```python
from build123d import *

# Parameters (mm, degrees)
SKETCH1_W           = 2.54
SKETCH1_H           = 2.54
BOSS_EXTRUDE1_DEPTH = 29.21
SKETCH2_OUTSIDE_W   = 10.426
SKETCH2_OUTSIDE_H   = 10.426
SKETCH2_OUTSIDE_W_2 = 1.905
SKETCH2_OUTSIDE_H_2 = 1.905
CUT_EXTRUDE1_DEPTH  = 11.43
FILLET1_R           = 1.27
SKETCH3_W           = 1.524
SKETCH3_H           = 16.51
BOSS_EXTRUDE2_DEPTH = 20.32
CUT_EXTRUDE2_DEPTH  = 38.147445726
CUT_EXTRUDE3_DEPTH  = 38.147445726


with BuildPart() as part:
    # Sketch1 → Boss-Extrude1 (new body)
    with BuildSketch(Plane(origin=(0, 0, 0), x_dir=(1, 0, 0), z_dir=(0, 1, 0))):
        with Locations((1.27, 1.27)):
            Rectangle(SKETCH1_W, SKETCH1_H)
    extrude(amount=BOSS_EXTRUDE1_DEPTH)

    # Sketch2 outside → Cut-Extrude1 (cut)
    with BuildSketch(Plane(origin=(0, 29.21, 0), x_dir=(1, 0, 0), z_dir=(0, 1, 0))):
        with Locations((1.27, 1.27)):
            Rectangle(SKETCH2_OUTSIDE_W, SKETCH2_OUTSIDE_H)
        with Locations((1.27, 1.27)):
            Rectangle(SKETCH2_OUTSIDE_W_2, SKETCH2_OUTSIDE_H_2, mode=Mode.SUBTRACT)
    extrude(amount=-CUT_EXTRUDE1_DEPTH, mode=Mode.SUBTRACT)

    # Fillet1
    fillet1_edges = [part.edges().sort_by_distance(p)[0] for p in [
        (1.27, 0, -2.54),
        (2.54, 0, -1.27),
        (1.27, 0, 0),
        (0, 0, -1.27),
    ]]
    fillet(fillet1_edges, radius=FILLET1_R - 0.0001)  # a hair under: the kernel refuses the full size

    # Sketch3 → Boss-Extrude2 (add)
    with BuildSketch(Plane(origin=(2.54, 0, 0), x_dir=(0, 0, -1), z_dir=(1, 0, 0))):
        with Locations((1.27, 9.525)):
            Rectangle(SKETCH3_W, SKETCH3_H)
    extrude(amount=BOSS_EXTRUDE2_DEPTH)

    # Sketch4 → Cut-Extrude2 (cut, through all)
    with BuildSketch(Plane.XY.offset(-0.508)):
        Polygon((2.54, 17.78), (22.86, 9.525), (22.86, 17.78), align=None)
    extrude(amount=-CUT_EXTRUDE2_DEPTH, mode=Mode.SUBTRACT)

    # Sketch5 → Cut-Extrude3 (cut, through all)
    with BuildSketch(Plane.XY.offset(-0.508)):
        Polygon((2.54, 1.27), (22.86, 9.525), (22.86, 1.27), align=None)
    extrude(amount=-CUT_EXTRUDE3_DEPTH, mode=Mode.SUBTRACT)


solid = part.part
```
The model under review builds one solid part; all positions refer to its coordinate system, in mm. A direction names the side the tool comes from. Round coordinates to 2 decimals unless told otherwise and drop trailing zeros. Write each loop counter-clockwise with the first axis right and the second up, starting at its lowest first coordinate (ties: lowest second). Pieces come first, ordered by that corner, then holes. Notation, with made-up numbers: (5, -39) -> (52, -39) arc R20 cw to (52, -11) -> close; hole circle Ø8 at (2.25, 81.5). An arc over 180 degrees is marked (long way). Use CSV: the item, a comma, the result in double quotes.
Q1. For faces 1 (the flat face through (1, 24, -2.222)), 2 (the flat face through (0.318, 24, -1)), 3 (the flat face through (10, 9, -0.508)), 4 (the flat face through (2.54, 9.41, -2.38)), list the 3-axis set-ups (+Z, -Z, +X, -X, +Y, -Y) from which the entire face can be reached by the end or side of a thin tool; tool diameter is ignored.
Checks:
face 1,"-Z, +X, -X, +Y"
face 2,"+Z, -Z, -X, +Y"
face 3,"+Z, +X, +Y, -Y"
face 4,"+X, +Y, -Y"
Q2. To check wall thickness, follow probe 1 along Z at (x, y) = (8.5, 4.75); probe 2 along X at (y, z) = (13.5, -2.4); probe 3 along X at (y, z) = (18.5, -1.8). State the ranges of each line that lie inside material, in increasing order. Write a range as [from, to].
Checks:
probe 1,"[-2.03, -0.51]"
probe 2,"[0, 2.54]"
probe 3,"[0.32, 2.22]"
Q3. For pin 1 Ø10 at (x, y) = (10, 13) entering from -Z; pin 2 Ø10 at (x, y) = (10, 16.5) entering from +Z; pin 3 Ø1 at (x, y) = (1, 26) entering from +Z; pin 4 Ø3 at (x, y) = (8, 17.5) entering from -Z, all flat-tipped, find the tip position at first contact; note any pin that passes through.
Checks:
pin 1,"z = -2.03"
pin 2,"z = -0.51"
pin 3,"z = -0.32"
pin 4,"through"
Q4. Consider section A-A (y = 17). Give the boundary of the cut face in (x, z).
Checks:
outline,"(0, -2.54) -> (2.54, -2.54) -> (2.54, -2.03) -> (4.46, -2.03) -> (4.46, -0.51) -> (2.54, -0.51) -> (2.54, 0) -> (0, 0) -> close"
Q5. Consider section C-C (x = 15.5). Give the boundary of the cut face in (y, z) (3 decimals), then the cut area to 3 significant figures.
Checks:
outline,"(6.535, -2.032) -> (12.515, -2.032) -> (12.515, -0.508) -> (6.535, -0.508) -> close"
area,"9.11 mm²"
Q6. Consider section D-D (y = 10.25). Give the boundary of the cut face in (x, z), then the cut area to 3 significant figures.
Checks:
outline,"(0, -2.54) -> (2.54, -2.54) -> (2.54, -2.03) -> (21.08, -2.03) -> (21.08, -0.51) -> (2.54, -0.51) -> (2.54, 0) -> (0, 0) -> close"
area,"34.7 mm²"
